```python
from build123d import *

# Parameters (mm, degrees)
BOSS_EXTRUDE1_DEPTH = 17


with BuildPart() as part:
    # Sketch2 → Boss-Extrude1 (new body)
    with BuildSketch(Plane.XY):
        with BuildLine():
            Line((35.613241121, -15.95389552), (37.863241121, -15.95389552))
            ThreePointArc((37.863241121, -15.95389552), (34.568192409, -7.998944231), (26.613241121, -4.70389552))
            Line((26.613241121, -4.70389552), (-51.886758879, -4.70389552))
            Line((-51.886758879, -4.70389552), (-51.886758879, -6.95389552))
            Line((-51.886758879, -6.95389552), (26.613241121, -6.95389552))
            ThreePointArc((26.613241121, -6.95389552), (32.977202152, -9.589934489), (35.613241121, -15.95389552))
        make_face()
    extrude(amount=BOSS_EXTRUDE1_DEPTH)


solid = part.part
```
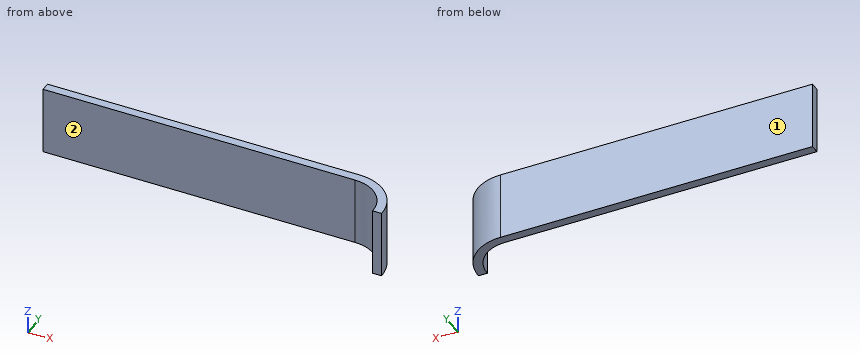
For this review, take the finished solid that the model builds, in its own axes (mm). Face numbers are marked on the shaded views. A direction names the side the tool comes from. Give positions to 0.01 mm unless a question says otherwise; leave off trailing zeros. Write each loop counter-clockwise with the first axis right and the second up, starting at its lowest first coordinate (ties: lowest second). Pieces come first, ordered by that corner, then holes.
Item 1: Take a section at B-B (x = 25). Give the boundary of the cut face in (y, z), and give its area (4 significant figures).
Item 2: Insertion check: P1, Ø6, axis at y = -12, z = 15, coming from the +X side; P2, Ø3, axis at y = -13.5, z = 13.5, coming from the -X side; P3, Ø1, axis at y = -9.5, z = 6, coming from the +X side; P4, Ø1.5, axis at y = -7.5, z = 2.5, coming from the -X side. Each pin has a flat end and moves straight along its axis. Give the tip position at first contact, or say it passes through.
Item 3: Machinability: for the marked faces 1 and 2, which of the approach directions +Z, -Z, +X, -X, +Y, -Y give a long, thin tool a straight path to every point of the face, cutting with its end or side? Answer none if there is none.
Item 4: Take a section at A-A (z = 5.5). Give the boundary of the cut face in (x, y), and give its area (3 significant figures).
Item 5: Wall thickness on probe 1 along Y at (x, z) = (-25, 12.75); probe 2 along X at (y, z) = (-13, 11.25); probe 3 along X at (y, z) = (-9.25, 9.5): over which ranges is each line inside the solid? List them lowest first.
Item 6: Take a section at C-C (y = -5.5). Give the boundary of the cut face in (x, z).
Established:
1. outline: (-6.95, 0) - (-4.7, 0) - (-4.7, 17) - (-6.95, 17) - close
1. area: 38.25 mm2
2. P1: stops at x = 37.82
2. P2: stops at x = 34.7
2. P3: stops at x = 36.16
2. P4: stops at x = -51.89
3. face 1: +Z, -Z, +X, -X, +Y
3. face 2: +Z, -Z, -X, -Y
4. outline: (-51.89, -6.95) - (26.61, -6.95) arc R9 cw to (35.61, -15.95) - (37.86, -15.95) arc R11.25 ccw to (26.61, -4.7) - (-51.89, -4.7) - close
4. area: 212 mm2
5. probe 1: y = -6.95 to -4.7
5. probe 2: x = 35.11 to 37.47
5. probe 3: x = 32.62 to 35.65
6. outline: (-51.89, 0) - (30.77, 0) - (30.77, 17) - (-51.89, 17) - close
